Can you work these out from the model? Positions are in its coordinate system, mm. A direction names the side the tool comes from. Round coordinates to 2 decimals unless told otherwise and drop trailing zeros. Write each loop counter-clockwise with the first axis right and the second up, starting at its lowest first coordinate (ties: lowest second). Pieces come first, ordered by that corner, then holes. Notation, with made-up numbers: (-28.5, -4.75) - (17.5, -4.75) arc R14 ccw to (17.5, 7.25) - close; hole circle Ø1 at (-33.75, -35). An arc over 180 degrees is marked (long way). One line per item, written item: value. Start each with the question number.
(1) If I drill on L1, parallel to Z at x = 10, y = 9; L2, parallel to Y at x = 23.5, z = 13; L3, parallel to Z at x = 4, y = 2.75, over which ranges is the centre line in solid material (lowest first)? Write a range as from..to.
(2) I'm going to push flat-ended pins straight in: pin 1 Ø1.5 at (x, z) = (2, 11) entering from -Y; pin 2 Ø2.5 at (x, y) = (3.5, 4) entering from +Z; pin 3 Ø5.5 at (x, z) = (24, 9.5) entering from -Y. Where does each tip first touch, or does it pass through?
(3) I want a section at B-B on x = 26.5. List the corners of the cut face in (y, z) for me, plus the area to 3 significant figures.
(4) Thinking about a two-plate mould opening in Z: for faces 1 (the face through (17, 12, 0)), 2 (the face through (22, 10, 10)), 3 (the face through (15.2, 20, 9.9)), which applies, +Z half, -Z half, draft (parallel to the pull), parting line (faces both ways), or undercut?
(5) I want a section at D-D on x = 13.75. List the corners of the cut face in (y, z) for me, plus the area to 3 significant figures.
(6) On a 3-axis mill with a long thin cutter (end or side, diameter ignored), from which of +Z, -Z, +X, -X, +Y, -Y can I reach the whole of each face in a straight line? I mean faces 4 (the face through (3, 5, 12.5)), 5 (the face through (10, 0, 4)), 6 (the face through (22, 5, 16)), 7 (the face through (16, 3, 2)), 8 (the face through (5, 12, 10)). Say none if no direction works.
from build123d import *

# Parameters (mm, degrees)
F1_DEPTH = 20
F2_R     = 9.99999
F4_DEPTH = 25
F5_R     = 5
F6_DEPTH = 20.001
F7_R     = 9.99999
F8_W     = 10
F8_H     = 5
F9_DEPTH = 30.001


# Not quite as in the source:
# - a fillet or chamfer is up to 0.001 mm smaller than in the source, because OpenCascade refuses the exact size


with BuildPart() as f1:
    # F0 (on Top) → F1 (new body)
    with BuildSketch(Plane.XY):
        Polygon((30, 20), (0, 20), (0, 0), (20, 0), (20, 5), (30, 5), align=None)
    extrude(amount=F1_DEPTH)

    # F2 (radius 10 in the source; OpenCascade refuses exactly that, so slightly less here)
    f2_edges = [f1.edges().sort_by_distance(p)[0] for p in [
        (0, 10, 20),
        (0, 10, 0),
    ]]
    fillet(f2_edges, radius=F2_R)

    # F3 (on Front) → F4 (cut)
    with BuildSketch(Plane.XZ):
        Polygon((30, 20), (25, 20), (30, 15), align=None)
        Polygon((30, 0), (30, 5), (25, 0), align=None)
    extrude(amount=-F4_DEPTH, mode=Mode.SUBTRACT)

    # F5 (on face) → F6 (cut, through all)
    with BuildSketch(Plane.XZ):
        with Locations((10, 10)):
            Circle(F5_R)
    extrude(amount=-F6_DEPTH, mode=Mode.SUBTRACT)

    # F7 (radius 10 in the source; OpenCascade refuses exactly that, so slightly less here)
    f7_edges = [f1.edges().sort_by_distance(p)[0] for p in [
        (20, 2.5, 20),
        (20, 2.5, 0),
    ]]
    fillet(f7_edges, radius=F7_R)

    # F8 (on Right) → F9 (cut, through all)
    with BuildSketch(Plane.YZ):
        with Locations((5, 10)):
            Rectangle(F8_W, F8_H)
    extrude(amount=F9_DEPTH, mode=Mode.SUBTRACT)


solid = f1.part
Established:
1. L1: 0..5, 15..20
1. L2: 5..20
1. L3: 2..7.5, 12.5..18
2. pin 1: y = 10
2. pin 2: z = 18.51
2. pin 3: y = 5
3. outline: (5, 1.5) - (20, 1.5) - (20, 18.5) - (5, 18.5) - (5, 12.5) - (10, 12.5) - (10, 7.5) - (5, 7.5) - close
3. area: 230 mm2
4. face 1: -Z half
4. face 2: undercut
4. face 3: draft
5. outline: (0, 0.73) - (5, 0.73) - (5, 0) - (20, 0) - (20, 6.69) - (0, 6.69) - close; (0, 13.31) - (20, 13.31) - (20, 20) - (5, 20) - (5, 19.27) - (0, 19.27) - close
5. area: 260 mm2
6. face 4: +X, -X, -Y
6. face 5: +Z, -Z, +X, -X, -Y
6. face 6: +Z, +X, -Y
6. face 7: -Z, +X, -Y
6. face 8: +Y, -Y
